```python
from build123d import *

# Parameters (mm, degrees)
BOSS_EXTRUDE1_DEPTH = 15.8
FILLET1_R           = 1
FILLET2_R           = 1
FILLET3_R           = 1
FILLET4_R           = 1
SKETCH3_R           = 2.85
BOSS_EXTRUDE2_DEPTH = 7.8
BOSS_EXTRUDE4_DEPTH = 15.8


with BuildPart() as part:
    # Sketch1 → Boss-Extrude1 (new body)
    with BuildSketch(Plane(origin=(0, 0, 0), x_dir=(1, 0, 0), z_dir=(0, 1, 0))):
        with BuildLine():
            Line((-0.8, -0.8), (-0.8, -2.102974084))
            ThreePointArc((-0.8, -2.102974084), (0, -2.25), (0.8, -2.102974084))
            Line((0.8, -2.102974084), (0.8, -0.8))
            Line((0.8, -0.8), (2.102974084, -0.8))
            ThreePointArc((2.102974084, -0.8), (2.25, 0), (2.102974084, 0.8))
            Line((2.102974084, 0.8), (0.8, 0.8))
            Line((0.8, 0.8), (0.8, 2.102974084))
            ThreePointArc((0.8, 2.102974084), (0, 2.25), (-0.8, 2.102974084))
            Line((-0.8, 2.102974084), (-0.8, 0.8))
            Line((-0.8, 0.8), (-2.102974084, 0.8))
            ThreePointArc((-2.102974084, 0.8), (-2.25, 0), (-2.102974084, -0.8))
            Line((-2.102974084, -0.8), (-0.8, -0.8))
        make_face()
    extrude(amount=BOSS_EXTRUDE1_DEPTH)

    # Fillet1
    fillet1_edges = [part.edges().sort_by_distance(p)[0] for p in [
        (-2.25, 0, 0),
    ]]
    fillet(fillet1_edges, radius=FILLET1_R)

    # Fillet2
    fillet2_edges = [part.edges().sort_by_distance(p)[0] for p in [
        (0, 0, 2.25),
    ]]
    fillet(fillet2_edges, radius=FILLET2_R)

    # Fillet3
    fillet3_edges = [part.edges().sort_by_distance(p)[0] for p in [
        (2.25, 0, 0),
    ]]
    fillet(fillet3_edges, radius=FILLET3_R)

    # Fillet4
    fillet4_edges = [part.edges().sort_by_distance(p)[0] for p in [
        (0, 0, -2.25),
    ]]
    fillet(fillet4_edges, radius=FILLET4_R)

    # Sketch3 → Boss-Extrude2 (add)
    with BuildSketch(Plane(origin=(0, 15.8, 0), x_dir=(1, 0, 0), z_dir=(0, 1, 0))):
        with Locations(Location((0, 0, 0), (0, 0, 270))):
            Circle(SKETCH3_R)
    extrude(amount=-BOSS_EXTRUDE2_DEPTH)

    # Sketch6 → Boss-Extrude4 (add)
    with BuildSketch(Plane(origin=(0, 15.8, 0), x_dir=(1, 0, 0), z_dir=(0, 1, 0))):
        with BuildLine():
            Line((-0.82856076, -0.791213071), (-0.82856076, -2.094187155))
            ThreePointArc((-0.82856076, -2.094187155), (-0.02856076, -2.241213071), (0.77143924, -2.094187155))
            Line((0.77143924, -2.094187155), (0.77143924, -0.791213071))
            Line((0.77143924, -0.791213071), (2.074413324, -0.791213071))
            ThreePointArc((2.074413324, -0.791213071), (2.22143924, 0.008786929), (2.074413324, 0.808786929))
            Line((2.074413324, 0.808786929), (0.77143924, 0.808786929))
            Line((0.77143924, 0.808786929), (0.77143924, 2.111761014))
            ThreePointArc((0.77143924, 2.111761014), (-0.02856076, 2.258786929), (-0.82856076, 2.111761014))
            Line((-0.82856076, 2.111761014), (-0.82856076, 0.808786929))
            Line((-0.82856076, 0.808786929), (-2.131534845, 0.808786929))
            ThreePointArc((-2.131534845, 0.808786929), (-2.27856076, 0.008786929), (-2.131534845, -0.791213071))
            Line((-2.131534845, -0.791213071), (-0.82856076, -0.791213071))
        make_face()
    extrude(amount=BOSS_EXTRUDE4_DEPTH)


solid = part.part
```
Verification items for the finished model (mm, model axes). A direction names the side the tool comes from. Give positions to 0.01 mm unless a question says otherwise; leave off trailing zeros. Order: outer loops, then holes, each group sorted by start corner. A loop starts at its lowest first (then second) coordinate and runs counter-clockwise, first axis right, second up. Notation, with made-up numbers: M 89.5,40.5 L 95.5,40.5 A15 ccw 95.5,57.5 Z; hole C 46.25,3 d7. An arc over 180 degrees is marked long. Answer in a Markdown table with one row per item. Add a question column.
Item 1: Section check A-A, the plane y = 4. Enter the section's corners in (x, z), and give its area (3 significant figures).
Item 2: Section check C-C, the plane z = 0. Enter the section's corners in (x, y).
Item 3: Gauge pin test, flat ends, axial feed: pin 1 (1 mm diameter, centred on y = 6, z = 1.5, fed in from +X); pin 2 (0.7 mm diameter, centred on x = 1.5, y = 21, fed in from -Z); pin 3 (0.7 mm diameter, centred on x = 1.5, y = 4.5, fed in from +Z). Record the tip position at first contact, or that the pin passes through.
Item 4: Section check B-B, the plane x = 0. Enter the section's corners in (y, z).
Item 5: Tool access check on faces 1 (the flat face through (0.8, 4, -1)), 2 (the cylindrical face through (0.01, 4.45, -2.25)), 3 (the flat face through (-1, 24, 0.791)), 4 (the flat face through (0.771, 24, -1)). Record the directions out of +Z, -Z, +X, -X, +Y, -Y that give a thin tool (end or side, any length) a straight path to the whole face; none if there is none.
Item 6: Scan lines: probe 1 along X at (y, z) = (19.5, -0.9); probe 2 along Z at (x, y) = (1.9, 27.5); probe 3 along X at (y, z) = (9.5, 0.2). Record each from-to range of solid material in increasing order. Write a range as from..to.
Filled sheet:
| question | item | result |
|---|---|---|
| 1 | outline | M -2.1,-0.8 L -0.8,-0.8 L -0.8,-2.1 A2.25 ccw 0.8,-2.1 L 0.8,-0.8 L 2.1,-0.8 A2.25 ccw 2.1,0.8 L 0.8,0.8 L 0.8,2.1 A2.25 ccw -0.8,2.1 L -0.8,0.8 L -2.1,0.8 A2.25 ccw Z |
| 1 | area | 11.5 mm^2 |
| 2 | outline | M -2.85,8 L -2.25,8 L -2.25,1 A1 ccw -1.25,0 L 1.25,0 A1 ccw 2.25,1 L 2.25,8 L 2.85,8 L 2.85,15.8 L 2.22,15.8 L 2.22,31.6 L -2.28,31.6 L -2.28,15.8 L -2.85,15.8 Z |
| 3 | pin 1 | stops at x = 0.8 |
| 3 | pin 2 | stops at z = -0.81 |
| 3 | pin 3 | stops at z = 0.8 |
| 4 | outline | M 0,-1.25 A1 ccw 1,-2.25 L 8,-2.25 L 8,-2.85 L 15.8,-2.85 L 15.8,-2.26 L 31.6,-2.26 L 31.6,2.24 L 15.8,2.24 L 15.8,2.85 L 8,2.85 L 8,2.25 L 1,2.25 A1 ccw 0,1.25 Z |
| 5 | face 1 | -Z, +X, -Y |
| 5 | face 2 | -Z, -Y |
| 5 | face 3 | +Z, -X, +Y |
| 5 | face 4 | -Z, +X, +Y |
| 6 | probe 1 | x = -0.83..0.77 |
| 6 | probe 2 | z = -0.81..0.79 |
| 6 | probe 3 | x = -2.84..2.84 |
